The listing builds one solid part. Answer for the finished solid, in the listing's coordinates (mm). Face numbers are marked on the shaded views. A direction names the side the tool comes from. Give positions to 0.01 mm unless a question says otherwise; leave off trailing zeros. Order: outer loops, then holes, each group sorted by start corner. A loop starts at its lowest first (then second) coordinate and runs counter-clockwise, first axis right, second up. Notation, with made-up numbers: (78.5, 42.25) -> (93.5, 42.25) arc R18 ccw to (93.5, 66.25) -> close; hole circle Ø9 at (27, 5.25). An arc over 180 degrees is marked (long way). Answer as a JSON object with one key per item and string values. Group by question number.
```python
from build123d import *

# Parameters (mm, degrees)
F0_W     = 10
F0_H     = 10
F1_DEPTH = 1
F0_R     = 2.5
F2_DEPTH = 2
F0_W_2   = 5
F0_H_2   = 5
F3_DEPTH = 5
F4_SIZE  = 5


with BuildPart() as f1:
    # F0 (on Top) → F1 (new body)
    with BuildSketch(Plane.XY):
        with Locations((-57.417053, 30.885033)):
            Rectangle(F0_W, F0_H)
    extrude(amount=F1_DEPTH)

    # F0 (on Top) → F2 (join)
    with BuildSketch(Plane.XY):
        Polygon((-42.417053, 35.885033), (-52.417053, 35.885033), (-52.417053, 25.885033), (-62.417053, 25.885033), (-62.417053, 15.885033), (-47.417053, 15.885033), (-47.417053, 20.885033), (-42.417053, 20.885033), align=None)
        with Locations((-57.417053, 20.885033)):
            Circle(F0_R, mode=Mode.SUBTRACT)
    extrude(amount=F2_DEPTH)

    # F0 (on Top) → F3 (join)
    with BuildSketch(Plane.XY):
        with Locations((-44.917053, 18.385033)):
            Rectangle(F0_W_2, F0_H_2)
    extrude(amount=F3_DEPTH)

    # F4
    f4_edges = [f1.edges().sort_by_distance(p)[0] for p in [
        (-42.417053, 35.885033, 1),
    ]]
    chamfer(f4_edges, length=F4_SIZE)


solid = f1.part
```
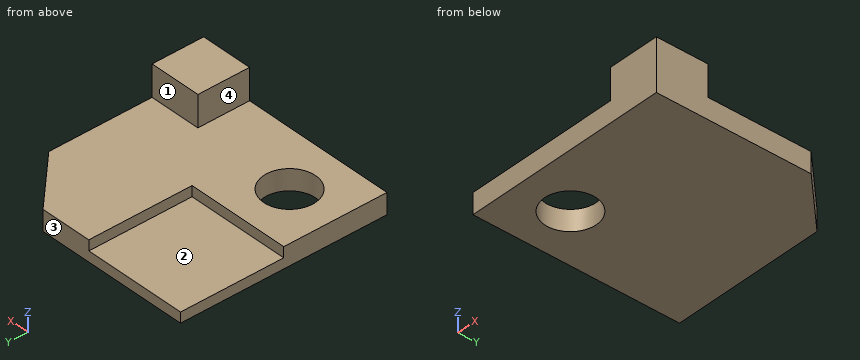
(1) A cutting plane is placed at B-B (x = -55.5). Determine the outline of the cut face in (y, z), and give its area (3 significant figures).
(2) Find the intervals of material crossed by line 1 along Z through (x, y) = (-47.5, 23.75); line 2 along Z through (x, y) = (-55.5, 33); line 3 along Y through (x, z) = (-46.5, 2.4), in increasing order. Write a range as [from, to].
(3) Flat-ended cylindrical pins translate along their axes: pin 1 Ø6 at (x, y) = (-57.42, 20.89) entering from +Z; pin 2 Ø1.5 at (y, z) = (29.5, 2.5) entering from +X; pin 3 Ø0.9 at (y, z) = (17.5, 3) entering from -X; pin 4 Ø0.8 at (x, z) = (-58.5, 1.5) entering from +Y. Find the tip coordinate at first contact, or state that the pin passes through.
(4) A cutting plane is placed at D-D (y = 29). Determine the outline of the cut face in (x, z).
(5) A cutting plane is placed at A-A (y = 19). Determine the outline of the cut face in (x, z), and give its area (3 significant figures).
(6) Which of the six approach directions +Z, -Z, +X, -X, +Y, -Y give full straight-line access (tool end or side, diameter ignored) to the marked faces 1, 2, 3 and 4?
(7) A cutting plane is placed at C-C (z = 0.65). Determine the outline of the cut face in (x, y).
Check sheet entries:
{
 "1": {"outline": "(15.89, 0) -> (19.28, 0) -> (19.28, 2) -> (15.89, 2) -> close; (22.49, 0) -> (35.89, 0) -> (35.89, 1) -> (25.89, 1) -> (25.89, 2) -> (22.49, 2) -> close", "area": "23.6 mm2"},
 "2": {"line 1": "z = [0, 2]", "line 2": "z = [0, 1]", "line 3": "y = [15.89, 20.89]"},
 "3": {"pin 1": "stops at z = 2", "pin 2": "stops at x = -42.42", "pin 3": "stops at x = -47.42", "pin 4": "stops at y = 25.89"},
 "4": {"outline": "(-62.42, 0) -> (-42.42, 0) -> (-42.42, 2) -> (-52.42, 2) -> (-52.42, 1) -> (-62.42, 1) -> close"},
 "5": {"outline": "(-62.42, 0) -> (-59.06, 0) -> (-59.06, 2) -> (-62.42, 2) -> close; (-55.77, 0) -> (-42.42, 0) -> (-42.42, 5) -> (-47.42, 5) -> (-47.42, 2) -> (-55.77, 2) -> close", "area": "48.4 mm2"},
 "6": {"face 1": "+Z, +X, -X, +Y", "face 2": "+Z, -X, +Y", "face 3": "+Z, -Z, +X, -X, +Y", "face 4": "+Z, -X, +Y, -Y"},
 "7": {"outline": "(-62.42, 15.89) -> (-42.42, 15.89) -> (-42.42, 30.89) -> (-47.42, 35.89) -> (-62.42, 35.89) -> close; hole circle Ø5 at (-57.42, 20.89)"}
}
